Read the model definition and answer for the solid it produces. Units are mm, in the model's axes. A direction names the side the tool comes from. Give positions to 0.01 mm unless a question says otherwise; leave off trailing zeros. Loops run counter-clockwise (first coordinate to the right, second up) from the corner with the lowest first, then second, coordinate; pieces in that order, holes last. Notation, with made-up numbers: (58.25, -39) - (74.25, -39) arc R21 ccw to (74.25, -29) - close; hole circle Ø9 at (81, -31.5). An arc over 180 degrees is marked (long way). Write each question's results on one line, items separated by ' | '. Start each with the question number.
Q1. The part is cut by section B-B, the plane y = 17. Write down the section's boundary in (x, z), plus the area to 3 significant figures.
Q2. Find the intervals of material crossed by line 1 (X direction, y = 4.6, z = 10); line 2 (X direction, y = 10.75, z = 28); line 3 (X direction, y = 13, z = 37), in increasing order. Write a range as from..to.
Q3. For faces 1 (the cylindrical face through (61.472, 18.739, -8.071)), 2 (the flat face through (-6.6, 12.6, 11.2)), determine the directions among +Z, -Z, +X, -X, +Y, -Y from which every point of the face is accessible in a straight line to the end or side of a thin tool.
Q4. The part is cut by section A-A, the plane z = 0. State how many separate pieces and enclosed holes the cut face has, plus the area to 3 significant figures.
Q5. The part is cut by section C-C, the plane y = 7.5. Write down the section's boundary in (x, z).
Q6. Given pin 1 (4 mm diameter, centred on y = 15, z = -1.5, fed in from +X); pin 2 (8 mm diameter, centred on y = 16.5, z = -17.5, fed in from +X); pin 3 (4 mm diameter, centred on y = 14.5, z = 20.5, fed in from -X), each flat-ended and moving along its own axis, determine where each tip first touches the part or whether it passes through.
```python
from build123d import *

# Parameters (mm, degrees)
SKETCH_1_R          = 62
EXTRUDE_1_DEPTH     = 20
SKETCH_3_R          = 9
CHAMFER_3_SIZE      = 1
CUT_EXTRUDE_2_DEPTH = 14
SKETCH_6_R          = 2
CUT_EXTRUDE_3_DEPTH = 90.933308624
CHAMFER_2_SIZE      = 1
CHAMFER_4_SIZE      = 2


with BuildPart() as part:
    # Эскиз1 → Бобышка-Вытянуть1 (new body)
    with BuildSketch(Plane(origin=(0, 0, 0), x_dir=(1, 0, 0), z_dir=(0, 1, 0))):
        with Locations(Location((0, 0, 0), (0, 0, 270))):
            Circle(SKETCH_1_R)
    extrude(amount=EXTRUDE_1_DEPTH)

    # Эскиз3 → Вырез-Повернуть2 (revolve, cut)
    with BuildSketch(Plane.XY, mode=Mode.PRIVATE) as cut_revolve_2_sk:
        with Locations((-65, 10)):
            Circle(SKETCH_3_R)
    revolve(cut_revolve_2_sk.sketch.rotate(Axis((0, 0, 0), (0, 1, 0)), 180), axis=Axis((0, 0, 0), (0, 1, 0)), mode=Mode.SUBTRACT)

    # Фаска3
    chamfer_3_edges = [part.edges().sort_by_distance(p)[0] for p in [
        (0, 0, -62),
    ]]
    chamfer(chamfer_3_edges, length=CHAMFER_3_SIZE)

    # Эскиз5 → Вырез-Вытянуть2 (cut)
    with BuildSketch(Plane(origin=(0, 20, 0), x_dir=(1, 0, 0), z_dir=(0, 1, 0))):
        Polygon((0, 15.011106999), (-13, 7.505553499), (-13, -7.505553499), (0, -15.011106999), (13, -7.505553499), (13, 7.505553499), align=None)
    extrude(amount=-CUT_EXTRUDE_2_DEPTH, mode=Mode.SUBTRACT)

    # Эскиз6 → Вырез-Вытянуть3 (cut, through all)
    with BuildSketch(Plane(origin=(0, 20, 0), x_dir=(1, 0, 0), z_dir=(0, 1, 0))):
        with Locations(Location((0, 10, 0), (0, 0, 270))):
            Circle(SKETCH_6_R)
        with Locations(Location((10, 0, 0), (0, 0, 270))):
            Circle(SKETCH_6_R)
        with Locations(Location((0, -10, 0), (0, 0, 270))):
            Circle(SKETCH_6_R)
        with Locations(Location((-10, 0, 0), (0, 0, 270))):
            Circle(SKETCH_6_R)
    extrude(amount=-CUT_EXTRUDE_3_DEPTH, mode=Mode.SUBTRACT)

    # Фаска2
    chamfer_2_edges = [part.edges().sort_by_distance(p)[0] for p in [
        (6.5, 20, -11.258330249),
        (-6.5, 20, -11.258330249),
        (-13, 20, 0),
        (-6.5, 20, 11.258330249),
        (6.5, 20, 11.258330249),
        (13, 20, 0),
        (0, 20, -62),
    ]]
    chamfer(chamfer_2_edges, length=CHAMFER_2_SIZE)

    # Фаска4
    chamfer_4_edges = [part.edges().sort_by_distance(p)[0] for p in [
        (0, 0, -12),
        (10, 0, -2),
        (0, 0, 8),
        (-10, 0, -2),
    ]]
    chamfer(chamfer_4_edges, length=CHAMFER_4_SIZE)


solid = part.part
```
Check sheet entries:
1) outline: circle Ø118.69 at (0, 0); hole (-13, -7.51) - (0, -15.01) - (13, -7.51) - (13, 7.51) - (0, 15.01) - (-13, 7.51) - close | area: 10,500 mm^2
2) line 1: x = -56.93..-2, 2..56.93 | line 2: x = -48.53..48.53 | line 3: x = -42.72..42.72
3) face 1: +Y, -Y | face 2: +Y
4) separate pieces: 3 | enclosed holes: 0 | area: 1,910 mm^2
5) outline: circle Ø112.71 at (0, 0); hole (-13, -7.51) - (0, -15.01) - (13, -7.51) - (13, 7.51) - (0, 15.01) - (-13, 7.51) - close
6) pin 1: stops at x = 59.32 | pin 2: stops at x = 60.39 | pin 3: stops at x = -55.2
